Can you work these out from the model? Positions are in its coordinate system, mm. Coordinates: 2 decimals unless noted, no trailing zeros. Order: outer loops, then holes, each group sorted by start corner. A loop starts at its lowest first (then second) coordinate and runs counter-clockwise, first axis right, second up. Notation, with made-up numbers: (17, -37) -> (56, -37) arc R35 cw to (56, -3) -> close; hole circle Ø10 at (-24, 36.5). An arc over 180 degrees is marked (long way). Return JSON: item names as keys, results as strings. Group by question number.
1) If we section it at D-D, the plane z = -3.5: Please give me the cut outline in (x, y), then the cut area to 3 significant figures.
2) If I drill on probe 1 along X at (y, z) = (21.5, 0); probe 2 along Z at (x, y) = (9, 15.5), over which ranges is the centre line in solid material (lowest first)? Write a range as from..to.
3) If we section it at B-B, the plane x = -6: Please give me the cut outline in (y, z), then the cut area to 3 significant figures.
4) If we section it at A-A, the plane z = 0: Please give me the cut outline in (x, y), then the cut area to 3 significant figures.
5) If we section it at C-C, the plane x = 0: Please give me the cut outline in (y, z).
6) For pin 1 (0.8 mm diameter, centred on x = -17.5, y = 47.5, fed in from -Z); pin 2 (2.5 mm diameter, centred on x = -19.5, z = -2, fed in from +Y); pin 3 (2.5 mm diameter, centred on x = -19.5, z = 1.5, fed in from -Y); pin 4 (5 mm diameter, centred on x = -10, z = 11, fed in from -Y), each with a flat end and sliding along its axis, tell me the tip position at first contact or that it passes through.
7) Thinking about a two-plate mould opening in Z: for faces 1 (the flat face through (-19, 48, 0)), 2 (the cylindrical face through (-9.139, 27.115, -14.334)), 3 (the cylindrical face through (13.094, 27.115, 10.04)), which applies, +Z half, -Z half, draft (parallel to the pull), parting line (faces both ways), or undercut?
Autodesk Inventor part; units mm, degrees
ref_plane "YZ Plane" through (0, 0, 0) normal (1, 0, 0) x (0, 1, 0)
ref_plane "XZ Plane" through (0, 0, 0) normal (0, 1, 0) x (-1, 0, 0)
ref_plane "XY Plane" through (0, 0, 0) normal (0, 0, 1) x (1, 0, 0)
sketch "Boceto1" plane through (0, 0, 0) normal (0, 1, 0) x (-1, 0, 0)
  circle A0 centre (0, 0) radius 16.5
  circle A1 centre (0, 0) radius 17
  dimension "d0" = 33
  dimension "d1" = 34
extrude "Extrusión1" add sketch "Boceto1" along normal blind 55
sketch "Boceto2" plane through (0, 0, 0) normal (1, 0, 0) x (0, 1, 0)
  line L0 (55, 5) -> (47, 5)
  line L1 (47, 5) -> (47, -5)
  line L2 (47, -5) -> (55, -5)
  line L3 (55, -5) -> (55, 5)
  line L4 (55, 16.5) -> (55, -16.5) construction
  line L5 (0, 16.5) -> (0, -16.5) construction
  point P0 (0, 0)
  point P1 (55, 0)
  dimension "d4" = 10
  dimension "d5" = 8
extrude "Extrusión2" cut sketch "Boceto2" against normal blind 55
sketch "Boceto3" plane through (-16.2481, 47, 5) normal (0, 1, 0) x (1, 0, 0)
  arc A0 (0, 10) -> (0, 0) centre (16.2481, 5) ccw construction
  line L0 (0.5239, 0) -> (0, 0) construction
  arc A1 (0.5239, 10) -> (0.5239, 0) centre (16.2481, 5) ccw construction
  line L1 (0.5239, 10) -> (0, 10) construction
  line L2 (0, 10) -> (-5, 10)
  line L3 (-5, 10) -> (-5, 0)
  line L4 (-5, 0) -> (0, 0)
  line L5 (0, 0) -> (0, 10)
  dimension "d8" = 5
  dimension "d9" = 10
extrude "Extrusión3" add sketch "Boceto3" along normal blind 1
properties part number "tuvo"
Result sheet:
{
 "1": {"outline": "(-21.25, 47) -> (-16.64, 47) -> (-16.64, 0) -> (-16.12, 0) -> (-16.12, 47) -> (-16.25, 47) -> (-16.25, 48) -> (-21.25, 48) -> close; (16.12, 0) -> (16.64, 0) -> (16.64, 55) -> (16.12, 55) -> close", "area": "57.2 mm2"},
 "2": {"probe 1": "x = -17..-16.5, 16.5..17", "probe 2": "z = -14.42..-13.83, 13.83..14.42"},
 "3": {"outline": "(0, -15.91) -> (55, -15.91) -> (55, -15.37) -> (0, -15.37) -> close; (0, 15.37) -> (55, 15.37) -> (55, 15.91) -> (0, 15.91) -> close", "area": "58.9 mm2"},
 "4": {"outline": "(-21.25, 47) -> (-17, 47) -> (-17, 0) -> (-16.5, 0) -> (-16.5, 47) -> (-16.25, 47) -> (-16.25, 48) -> (-21.25, 48) -> close; (16.5, 0) -> (17, 0) -> (17, 55) -> (16.5, 55) -> close", "area": "56.0 mm2"},
 "5": {"outline": "(0, -17) -> (55, -17) -> (55, -16.5) -> (0, -16.5) -> close; (0, 16.5) -> (55, 16.5) -> (55, 17) -> (0, 17) -> close"},
 "6": {"pin 1": "stops at z = -5", "pin 2": "stops at y = 48", "pin 3": "stops at y = 47", "pin 4": "stops at y = 0"},
 "7": {"face 1": "draft", "face 2": "parting line", "face 3": "undercut"}
}
